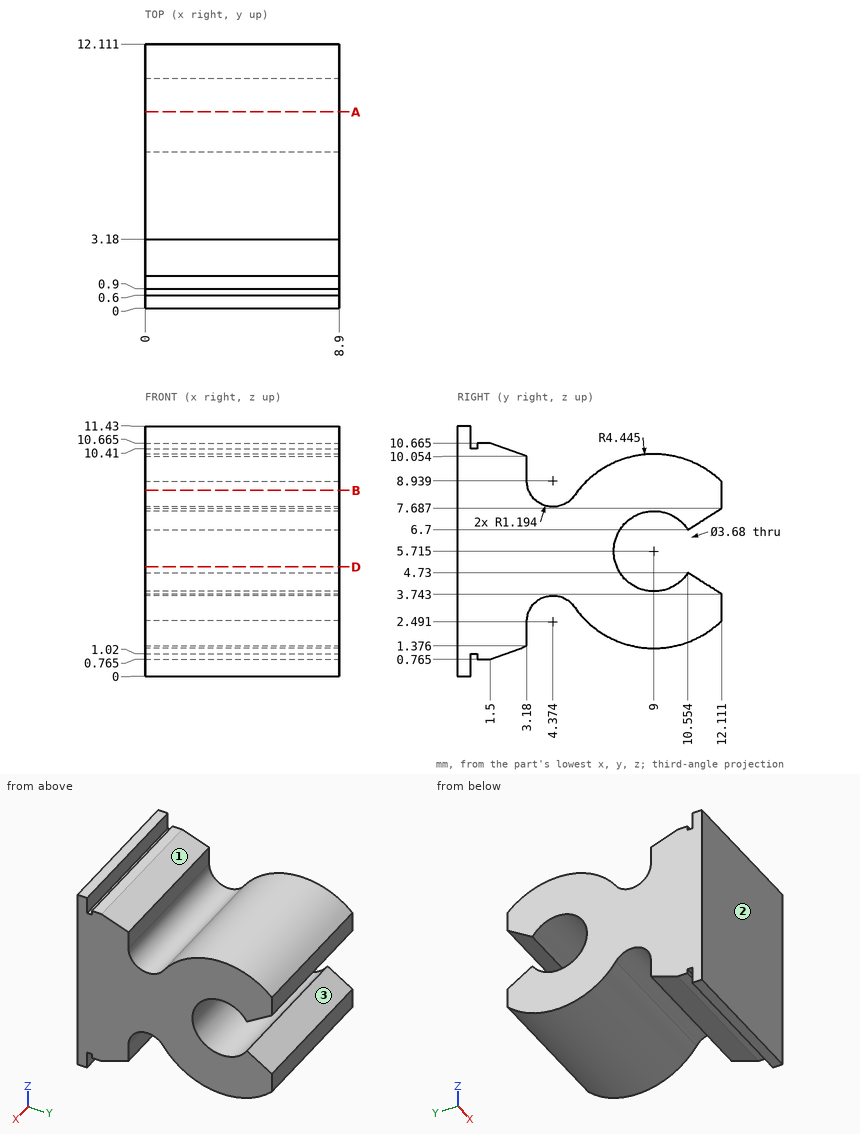
Here's the drawing with two shaded views (mm, measured from the low corner). I have some questions. A direction names the side the tool comes from. Coordinates: 2 decimals unless noted, no trailing zeros. Order: outer loops, then holes, each group sorted by start corner. A loop starts at its lowest first (then second) coordinate and runs counter-clockwise, first axis right, second up.
Q1. Please list where these lines run through material, in increasing order: L1, parallel to Z at x = 2.75, y = 9 (1 decimal); L2, parallel to Y at x = 7, z = 9.5; L3, parallel to Y at x = 8.75, z = 8.25.
Q2. Which directions (+Z, -Z, +X, -X, +Y, -Y) give clear straight access to the entire face, cutting with the end or side of a thin tool? Please do the marked faces 1, 2 and 3.
Q3. Suppose I cut it at A-A on y = 9. Please give me the cut outline in (x, z) (1 decimal).
Q4. Suppose I cut it at D-D on z = 5. Please give me the cut outline in (x, y) (1 decimal).
Q5. Will these pins go through, and if not, where does the flat tip stop? pin 1 (3 mm diameter, centred on y = 9, z = 5.715, fed in from +X); pin 2 (0.7 mm diameter, centred on x = 5.5, y = 1, fed in from +Z) (1 decimal); pin 3 (0.9 mm diameter, centred on x = 3, z = 1.5, fed in from +Y) (1 decimal); pin 4 (3 mm diameter, centred on x = 3.5, y = 9, fed in from +Z).
Q6. Suppose I cut it at B-B on z = 8.5. Please give me the cut outline in (x, y) (1 decimal).
Answer:
1. L1: z = 1.3 to 3.9, 7.6 to 10.2
1. L2: y = 0 to 3.18, 6.67 to 11.33
1. L3: y = 0 to 3.4, 5.35 to 12.11
2. face 1: +Z, +X, -X
2. face 2: +Z, -Z, +X, -X, -Y
2. face 3: +X, -X, +Y
3. outline: (0, 1.3) - (8.9, 1.3) - (8.9, 3.9) - (0, 3.9) - close; (0, 7.6) - (8.9, 7.6) - (8.9, 10.2) - (0, 10.2) - close
4. outline: (0, 0) - (8.9, 0) - (8.9, 7.3) - (0, 7.3) - close
5. pin 1: passes through
5. pin 2: stops at z = 10.7
5. pin 3: stops at y = 11.4
5. pin 4: stops at z = 10.16
6. outline: (0, 0) - (8.9, 0) - (8.9, 3.3) - (0, 3.3) - close; (0, 5.5) - (8.9, 5.5) - (8.9, 12.1) - (0, 12.1) - close
